Source: CAD feature listing. Evaluate the final solid. Frame: model axes, mm. A direction names the side the tool comes from. Give positions to 0.01 mm unless a question says otherwise; leave off trailing zeros. Loops run counter-clockwise (first coordinate to the right, second up) from the corner with the lowest first, then second, coordinate; pieces in that order, holes last. Notation, with made-up numbers: M 54,-21.5 L 78,-21.5 A6 cw 78,-17.5 Z; hole C -29.75,-4 d5. An arc over 180 degrees is marked long. Answer in a Markdown table with one row per item.
```python
from build123d import *

# Parameters (mm, degrees)
SKETCH1_R           = 1.5
SKETCH1_R_2         = 3
BOSS_EXTRUDE1_DEPTH = 5
SKETCH2_R           = 2.95
SKETCH2_R_2         = 1.5
BOSS_EXTRUDE2_DEPTH = 5


with BuildPart() as part:
    # Sketch1 → Boss-Extrude1 (new body)
    with BuildSketch(Plane.XY):
        with BuildLine():
            Line((-25, 6), (25, 6))
            ThreePointArc((25, 6), (31, 0), (25, -6))
            Line((25, -6), (-25, -6))
            ThreePointArc((-25, -6), (-31, 0), (-25, 6))
        make_face()
        with Locations((25, 0)):
            Circle(SKETCH1_R, mode=Mode.SUBTRACT)
        with Locations((-25, 0)):
            Circle(SKETCH1_R_2, mode=Mode.SUBTRACT)
    extrude(amount=BOSS_EXTRUDE1_DEPTH)

    # Sketch2 → Boss-Extrude2 (add)
    with BuildSketch(Plane.XY.offset(5)):
        with Locations((25, 0)):
            Circle(SKETCH2_R)
        with Locations((25, 0)):
            Circle(SKETCH2_R_2, mode=Mode.SUBTRACT)
    extrude(amount=BOSS_EXTRUDE2_DEPTH)


solid = part.part
```
1) Section A-A, the plane y = 0. Return loops of the section in (x, z).
Reply:
| item | result |
|---|---|
| outline | M -31,0 L -28,0 L -28,5 L -31,5 Z; M -22,0 L 23.5,0 L 23.5,10 L 22.05,10 L 22.05,5 L -22,5 Z; M 26.5,0 L 31,0 L 31,5 L 27.95,5 L 27.95,10 L 26.5,10 Z |
2) Pin query (flat end, axial travel): pin 1 Ø6 at (x, y) = (-9.5, -0.5) entering from +Z; pin 2 Ø2 at (y, z) = (0, 7) entering from +X; pin 3 Ø2 at (y, z) = (-2.5, 5) entering from -X. Return the tip coordinate at first contact, or that it passes through.
Reply:
| item | result |
|---|---|
| pin 1 | stops at z = 5 |
| pin 2 | stops at x = 27.95 |
| pin 3 | stops at x = -30.81 |
3) Section D-D, the plane z = 2. Return loops of the section in (x, y).
Reply:
| item | result |
|---|---|
| outline | M -25,-6 L 25,-6 A6 ccw 25,6 L -25,6 A6 ccw Z; hole C -25,0 d6; hole C 25,0 d3 |
4) Material intervals for L1, parallel to Y at x = -25, z = 1.05; L2, parallel to Y at x = 25, z = 2; L3, parallel to Z at x = -26, y = 4, sorted ascending.
Reply:
| item | result |
|---|---|
| L1 | y = -6 to -3, 3 to 6 |
| L2 | y = -6 to -1.5, 1.5 to 6 |
| L3 | z = 0 to 5 |
5) Section B-B, the plane z = 8.5. Return loops of the section in (x, y), then the cut area to 3 significant figures.
Reply:
| item | result |
|---|---|
| outline | C 25,0 d5.9; hole C 25,0 d3 |
| area | 20.3 mm² |
6) Section C-C, the plane x = -17. Return loops of the section in (y, z).
Reply:
| item | result |
|---|---|
| outline | M -6,0 L 6,0 L 6,5 L -6,5 Z |
7) Pull-direction query (Y, two-part tool) for faces 1 (the cylindrical face through (31, 0, 2)), 2 (the flat face through (26.3, -1.3, 10)), 3 (the cylindrical face through (-28, 0, 2)); classes: released by +Y, released by -Y, zero draft, split by the parting line, or undercut.
Reply:
| item | result |
|---|---|
| face 1 | split by the parting line |
| face 2 | zero draft |
| face 3 | undercut |
8) Set-up query: faces 4 (the cylindrical face through (27.814, 0.886, 7.465)), 5 (the cylindrical face through (-31, 0, 2)). Return all of +Z, -Z, +X, -X, +Y, -Y with unobstructed straight access to the full face (end or side cutting, diameter ignored); none if empty.
Reply:
| item | result |
|---|---|
| face 4 | +Z |
| face 5 | +Z, -Z, -X |
